The model under review builds one solid part; all positions refer to its coordinate system, in mm. A direction names the side the tool comes from. Coordinates: 2 decimals unless noted, no trailing zeros. Write each loop counter-clockwise with the first axis right and the second up, starting at its lowest first coordinate (ties: lowest second). Pieces come first, ordered by that corner, then holes. Notation, with made-up numbers: (75.5, -33.75) -> (81.5, -33.75) arc R22 cw to (81.5, -12.75) -> close; hole circle Ø4 at (24, 65). An arc over 180 degrees is marked (long way). Write each question's results on one line, items separated by ' | '.
```python
from build123d import *

# Parameters (mm, degrees)
F1_DEPTH = 19.05
F3_DEPTH = 6.35
F5_DEPTH = 0.508
F7_DEPTH = 19.05


with BuildPart() as f1:
    # F0 (on Front) → F1 (new body)
    with BuildSketch(Plane.XZ):
        with BuildLine():
            Line((29.9496520311, 63.0492046475), (26.6780648381, 69.4930180907))
            ThreePointArc((26.6780648381, 69.4930180907), (20.196677745, 54.5788891456), (16.5568571538, 38.7298725545))
            Line((16.5568571538, 38.7298725545), (16.690030694, 36.9986146688))
            Line((16.690030694, 36.9986146688), (13.6270336807, 35.6668755412))
            Line((13.6270336807, 35.6668755412), (13.8933807611, 44.5895195007))
            ThreePointArc((13.8933807611, 44.5895195007), (12.059862786, 49.3226978569), (8.1669082865, 52.579946816))
            ThreePointArc((8.1669082865, 52.579946816), (8.9030534245, 48.1186248362), (8.1669082865, 43.6573028564))
            ThreePointArc((8.1669082865, 43.6573028564), (5.3520163839, 36.253752533), (4.9707368016, 28.3423177898))
            ThreePointArc((4.9707368016, 28.3423177898), (6.7166015974, 24.6666402647), (8.6351158097, 21.0780538619))
            ThreePointArc((8.6351158097, 21.0780538619), (10.6419239697, 15.6995218737), (14.1597287729, 11.1629003659))
            ThreePointArc((14.1597287729, 11.1629003659), (15.0065668093, 13.1274904124), (14.1597287729, 15.092080459))
            Line((14.1597287729, 15.092080459), (14.1597287729, 15.8760100603))
            Line((14.1597287729, 15.8760100603), (14.5907411352, 16.6818480939))
            ThreePointArc((14.5907411352, 16.6818480939), (13.3602258193, 19.0818671101), (12.7488272265, 21.7087380588))
            Line((12.7488272265, 21.7087380588), (18.9269129187, 18.9074929804))
            ThreePointArc((18.9269129187, 18.9074929804), (20.5891941392, 12.5557803876), (24.337535724, 7.1652918123))
            Line((24.337535724, 7.1652918123), (25.5271047354, 9.0072061867))
            Line((25.5271047354, 9.0072061867), (25.9875822812, 8.0095026642))
            Line((25.9875822812, 8.0095026642), (32.2040431201, 18.4086412191))
            ThreePointArc((32.2040431201, 18.4086412191), (36.1728690985, 19.8478549134), (39.840310812, 21.9389759004))
            Line((39.840310812, 21.9389759004), (38.4588763118, 18.9842395484))
            ThreePointArc((38.4588763118, 18.9842395484), (38.7377638768, 18.2275381272), (39.4182056189, 17.7946705371))
            Line((39.4182056189, 17.7946705371), (37.4002235949, 14.7152889057))
            Line((37.4002235949, 14.7152889057), (37.8449037671, 13.7271098793))
            Line((37.8449037671, 13.7271098793), (39.5333245397, 14.955053106))
            ThreePointArc((39.5333245397, 14.955053106), (39.1304643178, 12.6593692531), (38.343757391, 10.4653881863))
            Line((38.343757391, 10.4653881863), (39.0344746411, 8.9304596186))
            ThreePointArc((39.0344746411, 8.9304596186), (43.5369991038, 14.6406633619), (45.7881577313, 21.5552449226))
            ThreePointArc((45.7881577313, 21.5552449226), (46.6985474779, 23.4097692807), (48.0521768332, 24.9704606831))
            ThreePointArc((48.0521768332, 24.9704606831), (47.9784626543, 33.30312196), (44.9055731297, 41.0488322377))
            ThreePointArc((44.9055731297, 41.0488322377), (44.1544418608, 45.7455441356), (44.9055731297, 50.4422560334))
            Line((44.9055731297, 50.4422560334), (42.9699420929, 49.2538958788))
            ThreePointArc((42.9699420929, 49.2538958788), (40.1761373605, 42.4912587379), (39.559867233, 35.2002494037))
            ThreePointArc((39.559867233, 35.2002494037), (37.8715608426, 36.3530467771), (35.9947867692, 37.1636264026))
            Line((35.9947867692, 37.1636264026), (34.1347455978, 53.3873215318))
            ThreePointArc((34.1347455978, 53.3873215318), (31.023684759, 57.7770885722), (29.9496520311, 63.0492046475))
        make_face()
    extrude(amount=F1_DEPTH)

    # F2 (on face) → F3 (cut)
    with BuildSketch(Plane.XZ.offset(19.05)):
        with BuildLine():
            Line((36.058422178, 35.5022437871), (34.1347455978, 53.3873215318))
            ThreePointArc((34.1347455978, 53.3873215318), (31.023684759, 57.7770885722), (29.9496520311, 63.0492046475))
            Line((29.9496520311, 63.0492046475), (26.6780648381, 69.4930180907))
            ThreePointArc((26.6780648381, 69.4930180907), (20.196677745, 54.5788891456), (16.5568571538, 38.7298725545))
            ThreePointArc((16.5568571538, 38.7298725545), (17.0958351547, 35.1595534204), (18.1488934904, 31.7057520151))
            Line((18.1488934904, 31.7057520151), (18.1488934904, 35.0895822048))
            ThreePointArc((18.1488934904, 35.0895822048), (19.0937254429, 36.5651386602), (20.1296713203, 37.9782170057))
            ThreePointArc((20.1296713203, 37.9782170057), (21.4851518176, 34.6808703775), (21.7803176492, 31.128026545))
            Line((21.7803176492, 31.128026545), (23.4309658408, 33.5214659572))
            Line((23.4309658408, 33.5214659572), (26.3196006417, 28.8171190768))
            ThreePointArc((26.3196006417, 28.8171190768), (28.572476319, 28.4980796307), (30.0335567445, 26.753809303))
            Line((30.0335567445, 26.753809303), (34.4077758491, 27.9917959124))
            Line((34.4077758491, 27.9917959124), (36.058422178, 35.5022437871))
        make_face()
        with BuildLine():
            ThreePointArc((27.7005694807, 17.765365541), (27.3434417277, 13.2052238558), (25.5271047354, 9.0072061867))
            Line((25.5271047354, 9.0072061867), (25.9875822812, 8.0095026642))
            Line((25.9875822812, 8.0095026642), (32.2040431201, 18.4086412191))
            ThreePointArc((32.2040431201, 18.4086412191), (29.9985149549, 17.7635037289), (27.7005694807, 17.765365541))
        make_face()
    extrude(amount=-F3_DEPTH, mode=Mode.SUBTRACT)

    # F4 (on face) → F5 (join)
    with BuildSketch(Plane.XZ.offset(19.05)):
        with BuildLine():
            ThreePointArc((46.2402813137, 25.7814861834), (45.2187335689, 34.5397157881), (43.6017140746, 43.207783252))
            ThreePointArc((43.6017140746, 43.207783252), (43.0662958477, 36.3634908572), (43.6017140746, 29.5191984624))
            ThreePointArc((43.6017140746, 29.5191984624), (43.6658279482, 26.2475841373), (43.2472340763, 23.0022259057))
            ThreePointArc((43.2472340763, 23.0022259057), (45.2061975799, 23.8938442422), (46.2402813137, 25.7814861834))
        make_face()
        with BuildLine():
            add(Edge.make_bspline(
                [(23.1004096568, 27.3739621043), (22.294183528, 27.387058336), (20.4669677334, 23.8183321525), (23.2573713599, 18.5786067922), (25.274701666, 23.8290656185), (23.8975818691, 27.3610129433), (23.1004096568, 27.3739621043)],
                knots=[0, 0, 0, 0, 0.2520256396, 0.5034254726, 0.7508046074, 1, 1, 1, 1], degree=3))
        make_face()
        with BuildLine():
            ThreePointArc((26.4196954668, 20.0969539583), (24.7008830261, 18.5573119841), (23.8514598459, 16.4117831737))
            ThreePointArc((23.8514598459, 16.4117831737), (23.9183277727, 13.0038753965), (24.8005911708, 9.7114723176))
            ThreePointArc((24.8005911708, 9.7114723176), (26.1535443213, 14.8194965183), (26.4196954668, 20.0969539583))
        make_face()
        with BuildLine():
            ThreePointArc((22.4556811154, 16.4117831737), (21.5251128707, 18.4763731071), (19.9432764202, 20.0969539583))
            ThreePointArc((19.9432764202, 20.0969539583), (20.8059126552, 14.7609071695), (22.7348357439, 9.7114723176))
            ThreePointArc((22.7348357439, 9.7114723176), (22.6477960375, 13.0638166167), (22.4556811154, 16.4117831737))
        make_face()
        with BuildLine():
            ThreePointArc((47.6991795003, 28.1513109803), (48.0318296747, 28.0236684218), (48.3848965621, 28.0715488384))
            ThreePointArc((48.3848965621, 28.0715488384), (48.1179191479, 32.5176082952), (46.9887144833, 36.8261600773))
            ThreePointArc((46.9887144833, 36.8261600773), (46.369528668, 36.3848095296), (46.1505949497, 35.6566272676))
            ThreePointArc((46.1505949497, 35.6566272676), (47.3623200822, 31.9942253821), (47.6991795003, 28.1513109803))
        make_face()
        with BuildLine():
            ThreePointArc((8.9119747281, 43.9040847123), (6.9184195013, 36.1498479724), (6.1123180203, 28.1841307878))
            ThreePointArc((6.1123180203, 28.1841307878), (6.8779842089, 26.8316177222), (8.073723875, 25.838771835))
            ThreePointArc((8.073723875, 25.838771835), (8.0540428558, 31.3970840751), (8.8405050337, 36.899510771))
            ThreePointArc((8.8405050337, 36.899510771), (9.1865848284, 40.3986312024), (8.9119747281, 43.9040847123))
        make_face()
        with BuildLine():
            ThreePointArc((5.3984993137, 31.2417112291), (5.7384809183, 35.2204489081), (6.927839946, 39.0324518085))
            Line((6.927839946, 39.0324518085), (6.1507176873, 39.1854316164))
            ThreePointArc((6.1507176873, 39.1854316164), (5.1668291163, 35.2690259496), (4.820222396, 31.2458264954))
            Line((4.820222396, 31.2458264954), (5.3984993137, 31.2417112291))
        make_face()
        Polygon((32.8636430204, 20.9054443985), (36.2221449614, 21.8757595867), (34.6921607852, 23.0699963868), (34.6921607852, 24.2642313242), (32.8636430204, 23.7044338137), align=None)
        with BuildLine():
            Line((14.1096655279, 26.0258354247), (13.9593891799, 22.9824855924))
            ThreePointArc((13.9593891799, 22.9824855924), (14.6970245146, 22.4682314443), (15.5936423689, 22.4001165479))
            Line((15.5936423689, 22.4001165479), (15.5936423689, 25.0865276903))
            Line((15.5936423689, 25.0865276903), (14.1096655279, 26.0258354247))
        make_face()
    extrude(amount=F5_DEPTH)

    # F6 (on face) → F7 (cut, through all)
    with BuildSketch(Plane.XZ.offset(19.05)):
        Polygon((36.058422178, 35.5022437871), (35.9947867692, 37.1636264026), (34.1347455978, 53.3873215318), align=None)
    extrude(amount=-F7_DEPTH, mode=Mode.SUBTRACT)


solid = f1.part
```
Q1. Add section A-A (x = 31). Write out the cut boundary in (y, z), plus the area to 3 significant figures.
Solution:
outline: (-19.05, 17.97) -> (-12.7, 17.97) -> (-12.7, 16.39) -> (0, 16.39) -> (0, 57.83) -> (-12.7, 57.83) -> (-12.7, 27.03) -> (-19.05, 27.03) -> close | area: 584 mm²
Q2. Draft analysis for pull direction X (two halves, no side actions). For faces 5 (the cylindrical face through (15.006, -9.392, 13.097)), 6 (the cylindrical face through (45.18, -19.3, 23.87)), 7 (the flat face through (26, 0, 32)), state which applies: pulls with the +X half, pulls with the -X half, needs draft (parallel to the pull), parting line crosses it, or undercut.
Solution:
face 5: undercut | face 6: pulls with the +X half | face 7: needs draft
Q3. Machinability: for faces 1 (the cylindrical face through (12.101, -9.392, 49.264)), 2 (the flat face through (5.4, -19.558, 35.5)), 3 (the cylindrical face through (20.786, -19.3, 14.834)), 4 (the cylindrical face through (19.08, -15.919, 36.545)), which of the approach directions +Z, -Z, +X, -X, +Y, -Y give a long, thin tool a straight path to every point of the face, cutting with its end or side? Answer none if there is none.
Solution:
face 1: +Z, +Y, -Y | face 2: +Z, -Z, +X, -X, -Y | face 3: -Z, -X, -Y | face 4: +Z, -Y
Q4. Clearance check with flat-ended pins moving along their axes: P1, Ø5, axis at x = 39.5, y = -6, coming from the -Z side; P2, Ø21.5, axis at x = 29.5, z = 42.5, coming from the -Y side; P3, Ø3, axis at y = -11, z = 43.5, coming from the -X side; P4, Ø1, axis at x = 15, z = 37.5, coming from the +Y side. State where each tip first meets the part, or that it passes through.
Solution:
P1: z = 8.93 | P2: y = -19.05 | P3: x = 7.3 | P4: through
Q5. Add section B-B (z = 65). Write out the cut boundary in (x, y), plus the area to 3 significant figures.
Solution:
outline: (24.38, -12.7) -> (28.96, -12.7) -> (28.96, 0) -> (24.38, 0) -> close | area: 58.2 mm²
Q6. For line 1 (X direction, y = -8.25, z = 49); line 2 (X direction, y = -9.5, z = 44.5); line 3 (Y direction, x = 40, z = 23), list the stretches that pass through material, from the lowest coordinate up. Write a range as from..to.
Solution:
line 1: 8.88..12.28, 18.56..34.61, 42.82..44.51 | line 2: 8.42..13.89, 17.53..35.09, 40.76..44.21 | line 3: -19.05..0
